from build123d import *

# Parameters (mm, degrees)
SKETCH1_W                      = 25
SKETCH1_H                      = 16
BOSS_EXTRUDE1_DEPTH            = 90
M4X0_7_TAPPED_HOLE1_D          = 3.3
M4X0_7_TAPPED_HOLE1_DEPTH      = 8
M4X0_7_TAPPED_HOLE1_TIP        = 0.991420021
M4X0_7_TAPPED_HOLE2_D          = 3.3
M4X0_7_TAPPED_HOLE2_DEPTH      = 12
M4X0_7_TAPPED_HOLE2_TIP        = 0.991420021
M4X0_7_TAPPED_HOLE3_D          = 3.3
M4X0_7_TAPPED_HOLE4_AT_2_COUNT = 2
M4X0_7_TAPPED_HOLE4_AT_2_PITCH = 55.578772926
M4X0_7_TAPPED_HOLE4_AT_3_COUNT = 2
M4X0_7_TAPPED_HOLE4_AT_3_PITCH = 55
M4X0_7_TAPPED_HOLE4_AT_4_COUNT = 2
M4X0_7_TAPPED_HOLE4_AT_4_PITCH = 8


with BuildPart() as part:
    # Sketch1 → Boss-Extrude1 (new body)
    with BuildSketch(Plane(origin=(0, 0, 0), x_dir=(1, 0, 0), z_dir=(0, 1, 0))):
        Rectangle(SKETCH1_W, SKETCH1_H)
    extrude(amount=BOSS_EXTRUDE1_DEPTH)

    # M4x0.7 Tapped Hole1
    with Locations(Plane(origin=(0, 90, 0), x_dir=(1, 0, 0), z_dir=(0, 1, 0))):
        with Locations((-7.5, 0), (7.5, 0)):
            Hole(M4X0_7_TAPPED_HOLE1_D / 2, depth=M4X0_7_TAPPED_HOLE1_DEPTH)
            with Locations((0, 0, -(M4X0_7_TAPPED_HOLE1_DEPTH + M4X0_7_TAPPED_HOLE1_TIP / 2))):  # 118° drill point
                Cone(0, M4X0_7_TAPPED_HOLE1_D / 2, M4X0_7_TAPPED_HOLE1_TIP, mode=Mode.SUBTRACT)

    # M4x0.7 Tapped Hole2
    with Locations(Plane(origin=(0, 0, 0), x_dir=(-1, 0, 0), z_dir=(0, -1, 0))):
        with Locations((-7.5, 0), (7.5, 0)):
            Hole(M4X0_7_TAPPED_HOLE2_D / 2, depth=M4X0_7_TAPPED_HOLE2_DEPTH)
            with Locations((0, 0, -(M4X0_7_TAPPED_HOLE2_DEPTH + M4X0_7_TAPPED_HOLE2_TIP / 2))):  # 118° drill point
                Cone(0, M4X0_7_TAPPED_HOLE2_D / 2, M4X0_7_TAPPED_HOLE2_TIP, mode=Mode.SUBTRACT)

    # M4x0.7 Tapped Hole3 (through all)
    with Locations(Plane(origin=(0, 0, -8), x_dir=(-1, 0, 0), z_dir=(0, 0, -1))):
        with Locations((0, 20), (0, 65), (15, 65), (15, 20)):
            Hole(M4X0_7_TAPPED_HOLE3_D / 2)

    # Sketch13 → M4x0.7 Tapped Hole4 (revolve, cut)
    with BuildSketch(Plane(origin=(-12.5, 17.5, 4), x_dir=(0, 0, 1), z_dir=(0, 1, 0))):
        Polygon((0, 0), (0, 8.991420021), (1.65, 8), (1.65, 0), align=None)
    m4x0_7_tapped_hole4 = revolve(axis=Axis((-18.85, 17.5, 4), (1, 0, 0)), mode=Mode.SUBTRACT)

    # M4x0.7 Tapped Hole4 at 2: M4x0.7 Tapped Hole4 ×2
    with Locations(*[Vector(0, 0.9895864392845114, -0.14393984571411075) * (i * M4X0_7_TAPPED_HOLE4_AT_2_PITCH) for i in range(1, M4X0_7_TAPPED_HOLE4_AT_2_COUNT)]):
        add(m4x0_7_tapped_hole4, mode=Mode.SUBTRACT)

    # M4x0.7 Tapped Hole4 at 3: M4x0.7 Tapped Hole4 ×2
    with Locations(*[(0, i * M4X0_7_TAPPED_HOLE4_AT_3_PITCH, 0) for i in range(1, M4X0_7_TAPPED_HOLE4_AT_3_COUNT)]):
        add(m4x0_7_tapped_hole4, mode=Mode.SUBTRACT)

    # M4x0.7 Tapped Hole4 at 4: M4x0.7 Tapped Hole4 ×2
    with Locations(*[(0, 0, -i * M4X0_7_TAPPED_HOLE4_AT_4_PITCH) for i in range(1, M4X0_7_TAPPED_HOLE4_AT_4_COUNT)]):
        add(m4x0_7_tapped_hole4, mode=Mode.SUBTRACT)

    # Mirror1: M4x0.7 Tapped Hole4 across plane
    add(m4x0_7_tapped_hole4.mirror(Plane(origin=(0, 0, 0), x_dir=(0, 0, 1), z_dir=(1, 0, 0))), mode=Mode.SUBTRACT)

    # Mirror1 copy 1 sketch → Mirror1 copy 1 (revolve, cut)
    with BuildSketch(Plane(origin=(12.5, 72.5, -4), x_dir=(0, 0, 1), z_dir=(0, 1, 0))):
        Polygon((0, 0), (0, -8.991420021), (1.65, -8), (1.65, 0), align=None)
    revolve(axis=Axis((18.85, 72.5, -4), (1, 0, 0)), mode=Mode.SUBTRACT)

    # Mirror1 copy 2 sketch → Mirror1 copy 2 (revolve, cut)
    with BuildSketch(Plane(origin=(12.5, 72.5, 4), x_dir=(0, 0, 1), z_dir=(0, 1, 0))):
        Polygon((0, 0), (0, -8.991420021), (1.65, -8), (1.65, 0), align=None)
    revolve(axis=Axis((18.85, 72.5, 4), (1, 0, 0)), mode=Mode.SUBTRACT)

    # Mirror1 copy 3 sketch → Mirror1 copy 3 (revolve, cut)
    with BuildSketch(Plane(origin=(12.5, 17.5, -4), x_dir=(0, 0, 1), z_dir=(0, 1, 0))):
        Polygon((0, 0), (0, -8.991420021), (1.65, -8), (1.65, 0), align=None)
    revolve(axis=Axis((18.85, 17.5, -4), (1, 0, 0)), mode=Mode.SUBTRACT)


solid = part.part
Part model, mm, in its own coordinate system. A direction names the side the tool comes from. Give positions to 0.01 mm unless a question says otherwise; leave off trailing zeros. Write each loop counter-clockwise with the first axis right and the second up, starting at its lowest first coordinate (ties: lowest second). Pieces come first, ordered by that corner, then holes.
1) Two-plate mould, pull along X, no slides. Class faces 5 (the face through (9.15, 85.94, -0.07)), 6 (the face through (0, 90, 0)), 7 (the face through (-3.68, 17.22, 3.96)), 8 (the face through (12.5, 44, 0)): released by +X, released by -X, zero draft, split by the parting line, or undercut.
Resolved:
face 5: undercut
face 6: zero draft
face 7: released by -X
face 8: released by +X
2) Cut at A-A on x = 11. Write the cut outline in (y, z), then the cut area to 3 significant figures.
Resolved:
outline: (0, -8) - (90, -8) - (90, 8) - (0, 8) - close; hole circle Ø3.3 at (17.5, -4); hole circle Ø3.3 at (17.5, 4); hole circle Ø3.3 at (72.5, -4); hole circle Ø3.3 at (72.5, 4)
area: 1,410 mm2
3) Pin check, flat tips, straight feed: pin 1 (2 mm diameter, centred on y = 72.5, z = -4, fed in from -X); pin 2 (2.5 mm diameter, centred on y = 17.5, z = 4, fed in from +X); pin 3 (3 mm diameter, centred on y = 72.5, z = 4, fed in from -X). Stop position of each tip, or through.
Resolved:
pin 1: stops at x = -4.11
pin 2: stops at x = 4.26
pin 3: stops at x = -4.41
4) Probe L1, parallel to Y at x = 8.25, z = -3.75; L2, parallel to Y at x = 7.5, z = 5.5; L3, parallel to Z at x = -10.25, y = 17.5. List the from-to ranges inside material, lowest first.
Resolved:
L1: y = 0 to 15.87, 19.13 to 70.87, 74.13 to 90
L2: y = 0 to 16.81, 18.19 to 71.81, 73.19 to 90
L3: z = -8 to -5.65, -2.35 to 2.35, 5.65 to 8
5) Which spindle directions (+Z, -Z, +X, -X, +Y, -Y) get a long thin tool onto all of the face, cutting with end or side? Do faces 1 (the face through (8.6, 74.1, -4.4)), 2 (the face through (-5.85, 85.94, -0.07)), 3 (the face through (-8.6, 74.1, 3.6)), 4 (the face through (-0.4, 63.4, 0.1)). Say none if no direction does.
Resolved:
face 1: +X
face 2: +Y
face 3: -X
face 4: +Z, -Z
